from build123d import *

# Parameters (mm, degrees)
BOSS_EXTRU_1_DEPTH = 5


with BuildPart() as part:
    # Esquisse1 → Boss.-Extru.1 (new body)
    with BuildSketch(Plane.XY):
        with BuildLine():
            Line((50, 0), (50, 10))
            Line((50, 10), (15, 10))
            Line((15, 10), (15, 64.203101523))
            Line((15, 64.203101523), (32.561057994, 64.203101523))
            Line((32.561057994, 64.203101523), (32.561057994, 84.294650344))
            Line((32.561057994, 84.294650344), (5, 84.294650344))
            Line((5, 84.294650344), (5, 60.912399745))
            Line((5, 60.912399745), (0, 60.912399745))
            Line((0, 60.912399745), (0, 55.912399745))
            ThreePointArc((0, 55.912399745), (6.66837561, 35.361996844), (0, 14.811593943))
            Line((0, 14.811593943), (10, 0))
            Line((10, 0), (50, 0))
        make_face()
    extrude(amount=BOSS_EXTRU_1_DEPTH)


solid = part.part
Verification items for the finished model (mm, model axes). A direction names the side the tool comes from. Coordinates: 2 decimals unless noted, no trailing zeros. Order: outer loops, then holes, each group sorted by start corner. A loop starts at its lowest first (then second) coordinate and runs counter-clockwise, first axis right, second up. Notation, with made-up numbers: M -4.75,18.25 L 11.25,18.25 A16 ccw 11.25,32.25 Z; hole C 58,82 d9. An arc over 180 degrees is marked long. Return JSON: item names as keys, results as strings.
1) Gauge pin test, flat ends, axial feed: pin 1 (1 mm diameter, centred on x = 31, z = 3.5, fed in from -Y); pin 2 (2.5 mm diameter, centred on x = 36, z = 3.5, fed in from +Y); pin 3 (2.5 mm diameter, centred on y = 75.5, z = 2.5, fed in from +X). Record the tip position at first contact, or that the pin passes through.
Answer list:
{"pin 1": "y = 0", "pin 2": "y = 10", "pin 3": "x = 32.56"}
2) Access from +Z, -Z, +X, -X, +Y, -Y to the whole of each face (thin tool, end or side, straight path). Record for faces 1 (the flat face through (50, 5, 2)), 2 (the flat face through (5, 73, 2)), 3 (the flat face through (0, 58, 2)), 4 (the flat face through (15, 37, 2)), 5 (the flat face through (32.561, 74, 2)).
Answer list:
{"face 1": "+Z, -Z, +X, +Y, -Y", "face 2": "+Z, -Z, -X, +Y", "face 3": "+Z, -Z, -X, +Y, -Y", "face 4": "+Z, -Z, +X", "face 5": "+Z, -Z, +X, +Y"}
3) Thickness scan on L1, parallel to Y at x = 23, z = 3.5; L2, parallel to Y at x = 37.5, z = 3.5; L3, parallel to X at y = 71.5, z = 1.05. Record the ranges inside material, lowest first. Write a range as [from, to].
Answer list:
{"L1": "[0, 10], [64.2, 84.29]", "L2": "[0, 10]", "L3": "[5, 32.56]"}
4) Release check for a two-part mould opening along Y. For faces 6 (the flat face through (19, 84.295, 2)), 7 (the flat face through (14, 43, 0)), 8 (the cylindrical face through (6.667, 35.669, 2.465)) record: +Y half, -Y half, draft (parallel to the pull), parting line (faces both ways), or undercut.
Answer list:
{"face 6": "+Y half", "face 7": "draft", "face 8": "undercut"}
5) Cross-section at C-C, the plane y = 57.5. Record the boundary of the cut face in (x, z).
Answer list:
{"outline": "M 0,0 L 15,0 L 15,5 L 0,5 Z"}
6) Cross-section at A-A, the plane x = 26. Record the boundary of the cut face in (y, z), and give its area (3 significant figures).
Answer list:
{"outline": "M 0,0 L 10,0 L 10,5 L 0,5 Z; M 64.2,0 L 84.29,0 L 84.29,5 L 64.2,5 Z", "area": "150 mm2"}
7) Cross-section at D-D, the plane x = 38.5. Record the boundary of the cut face in (y, z).
Answer list:
{"outline": "M 0,0 L 10,0 L 10,5 L 0,5 Z"}
8) Cross-section at B-B, the plane z = 2.45. Record the boundary of the cut face in (x, y), and give its area (3 significant figures).
Answer list:
{"outline": "M 0,14.81 L 10,0 L 50,0 L 50,10 L 15,10 L 15,64.2 L 32.56,64.2 L 32.56,84.29 L 5,84.29 L 5,60.91 L 0,60.91 L 0,55.91 A35 cw Z", "area": "1,590 mm2"}
